For this review, use the dimensioned drawing (mm, ordinates from the lowest corner) and the shaded views. A direction names the side the tool comes from. Coordinates: 2 decimals unless noted, no trailing zeros. Write each loop counter-clockwise with the first axis right and the second up, starting at its lowest first coordinate (ties: lowest second). Pieces come first, ordered by that corner, then holes. Notation, with made-up numbers: (31.5, 52.25) - (62.5, 52.25) arc R21 ccw to (62.5, 89.25) - close; hole circle Ø11 at (73, -39). An arc over 180 degrees is marked (long way). One line per item, written item: value.
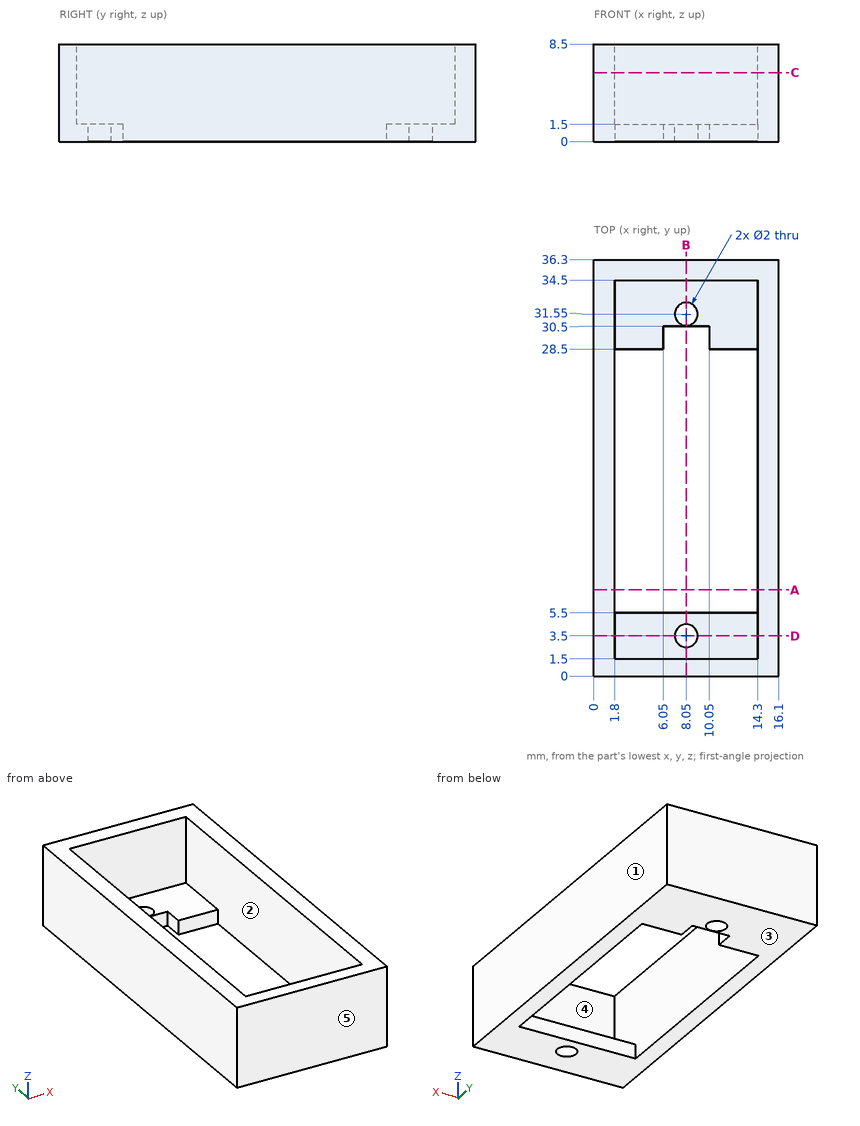
1. Consider section D-D, the plane y = 3.5. Write out the cut boundary in (x, z).
Answer block:
outline: (0, 0) - (7.05, 0) - (7.05, 1.5) - (1.8, 1.5) - (1.8, 8.5) - (0, 8.5) - close; (9.05, 0) - (16.1, 0) - (16.1, 8.5) - (14.3, 8.5) - (14.3, 1.5) - (9.05, 1.5) - close
2. Consider section C-C, the plane z = 6. Write out the cut boundary in (x, y), then the cut area to 3 significant figures.
Answer block:
outline: (0, 0) - (16.1, 0) - (16.1, 36.3) - (0, 36.3) - close; hole (1.8, 1.5) - (14.3, 1.5) - (14.3, 34.5) - (1.8, 34.5) - close
area: 172 mm^2
3. Mouldability with a two-part tool opening along X and no side actions: class the marked faces 1, 2 and 3 as released by +X, released by -X, zero draft, split by the parting line, or undercut.
Answer block:
face 1: released by +X
face 2: undercut
face 3: zero draft
4. Consider section B-B, the plane x = 8.05. Write out the cut boundary in (y, z).
Answer block:
outline: (0, 0) - (2.5, 0) - (2.5, 1.5) - (1.5, 1.5) - (1.5, 8.5) - (0, 8.5) - close; (4.5, 0) - (5.5, 0) - (5.5, 1.5) - (4.5, 1.5) - close; (30.5, 0) - (30.55, 0) - (30.55, 1.5) - (30.5, 1.5) - close; (32.55, 0) - (36.3, 0) - (36.3, 8.5) - (34.5, 8.5) - (34.5, 1.5) - (32.55, 1.5) - close
5. Insertion check: pin 1 Ø1.8 at (x, y) = (9, 32.5) entering from +Z. The pin has a flat end and moves straight along its axis. Give the tip position at first contact, or say it passes through.
Answer block:
pin 1: stops at z = 1.5
6. For the marked faces 4 and 5, list the 3-axis set-ups (+Z, -Z, +X, -X, +Y, -Y) from which the entire face can be reached by the end or side of a thin tool; tool diameter is ignored.
Answer block:
face 4: +Z
face 5: +Z, -Z, +X, -X, -Y
7. Wall thickness on line 1 along Y through (x, z) = (11, 5); line 2 along X through (y, z) = (21, 3.75); line 3 along Z through (x, y) = (2.25, 32): over which ranges is each line inside the solid? List them lowest first.
Answer block:
line 1: y = 0 to 1.5, 34.5 to 36.3
line 2: x = 0 to 1.8, 14.3 to 16.1
line 3: z = 0 to 1.5
8. Consider section A-A, the plane y = 7.5. Write out the cut boundary in (x, z), then the cut area to 3 significant figures.
Answer block:
outline: (0, 0) - (1.8, 0) - (1.8, 8.5) - (0, 8.5) - close; (14.3, 0) - (16.1, 0) - (16.1, 8.5) - (14.3, 8.5) - close
area: 30.6 mm^2
